The model under review builds one solid part; all positions refer to its coordinate system, in mm. Round coordinates to 2 decimals unless told otherwise and drop trailing zeros. Loops run counter-clockwise (first coordinate to the right, second up) from the corner with the lowest first, then second, coordinate; pieces in that order, holes last. Notation, with made-up numbers: (26.25, -8) - (44.25, -8) arc R13 ccw to (44.25, -4) - close; hole circle Ø5 at (36, 58). An arc over 180 degrees is marked (long way). Answer as CSV lines item,"result".
from build123d import *

# Parameters (mm, degrees)
F0_R     = 47.659552
F2_DEPTH = 101.6
F1_R     = 13.037105
F3_DEPTH = 101.6
F4_R     = 8.24229
F5_DEPTH = 101.6


with BuildPart() as f2:
    # F0 (on Top) → F2 (new body)
    with BuildSketch(Plane.XY):
        Circle(F0_R)
    extrude(amount=F2_DEPTH)

    # F1 (on face) → F3 (join)
    with BuildSketch(Plane.XY):
        Circle(F1_R)
    extrude(amount=F3_DEPTH)

    # F4 (on face) → F5 (cut)
    with BuildSketch(Plane(origin=(0, 0, 0), x_dir=(1, 0, 0), z_dir=(0, 0, -1))):
        Circle(F4_R)
    extrude(amount=-F5_DEPTH, mode=Mode.SUBTRACT)


solid = f2.part
1. Take a section at D-D (y = 16). State the section outline as (x, z) points.
Numbers:
outline,"(-44.89, 0) - (44.89, 0) - (44.89, 101.6) - (-44.89, 101.6) - close"
2. Take a section at B-B (y = 6). State the section outline as (x, z) points, plus the area to 3 significant figures.
Numbers:
outline,"(-47.28, 0) - (-5.65, 0) - (-5.65, 101.6) - (-47.28, 101.6) - close; (5.65, 0) - (47.28, 0) - (47.28, 101.6) - (5.65, 101.6) - close"
area,"8,460 mm²"
3. Wall thickness on probe 1 along Y at (x, z) = (0, 67); probe 2 along X at (y, z) = (-28, 87); probe 3 along Y at (x, z) = (7.5, 96): over which ranges is each line inside the solid? List them lowest first.
Numbers:
probe 1,"y = -47.66 to -8.24, 8.24 to 47.66"
probe 2,"x = -38.57 to 38.57"
probe 3,"y = -47.07 to -3.42, 3.42 to 47.07"
4. Clearance check with flat-ended pins moving along their axes: pin 1 (10 mm diameter, centred on x = 14.5, z = 52, fed in from -Y); pin 2 (2 mm diameter, centred on x = 35.5, z = 52, fed in from +Y); pin 3 (1.5 mm diameter, centred on y = 6, z = 17.5, fed in from +X). State where each tip first meets the part, or that it passes through.
Numbers:
pin 1,"stops at y = -46.7"
pin 2,"stops at y = 32.88"
pin 3,"stops at x = 47.37"
5. Take a section at A-A (x = 0). State the section outline as (y, z) points, plus the area to 3 significant figures.
Numbers:
outline,"(-47.66, 0) - (-8.24, 0) - (-8.24, 101.6) - (-47.66, 101.6) - close; (8.24, 0) - (47.66, 0) - (47.66, 101.6) - (8.24, 101.6) - close"
area,"8,010 mm²"
6. Take a section at C-C (z = 92.5). State the section outline as (x, y) points.
Numbers:
outline,"circle Ø95.32 at (0, 0); hole circle Ø16.48 at (0, 0)"
7. Draft analysis for pull direction X (two halves, no side actions). For faces 1 (the face through (-35.13, 32.21, 50.09)), 2 (the face through (-1.787, 8.046, 50.089)), 3 (the face through (-1, -10, 101.6)), state which applies: +X half, -X half, draft (parallel to the pull), parting line (faces both ways), or undercut.
Numbers:
face 1,"parting line"
face 2,"undercut"
face 3,"draft"
